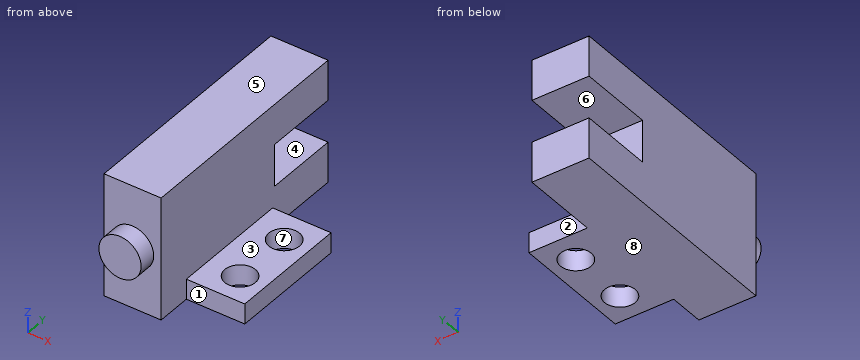
from build123d import *

# Parameters (mm, degrees)
SKETCH_1_W          = 6.5
SKETCH_1_H          = 14
EXTRUDE_1_DEPTH     = 26.5
SKETCH_2_W          = 6.5
SKETCH_2_H          = 4.8
CUT_EXTRUDE_1_DEPTH = 8.5
SKETCH_3_W          = 2.3
SKETCH_3_H          = 13.7
EXTRUDE_2_DEPTH     = 6.65
SKETCH_4_R          = 1.75
CUT_EXTRUDE_2_DEPTH = 6.65
SKETCH_5_R          = 2.4
EXTRUDE_3_DEPTH     = 2


with BuildPart() as part:
    # 草图1 → 凸台-拉伸1 (new body)
    with BuildSketch(Plane(origin=(0, 0, 0), x_dir=(1, 0, 0), z_dir=(0, 1, 0))):
        with Locations((3.25, 7)):
            Rectangle(SKETCH_1_W, SKETCH_1_H)
    extrude(amount=EXTRUDE_1_DEPTH)

    # 草图2 → 切除-拉伸1 (cut)
    with BuildSketch(Plane(origin=(0, 26.5, 0), x_dir=(1, 0, 0), z_dir=(0, 1, 0))):
        with Locations((3.25, 7)):
            Rectangle(SKETCH_2_W, SKETCH_2_H)
    extrude(amount=-CUT_EXTRUDE_1_DEPTH, mode=Mode.SUBTRACT)

    # 草图3 → 凸台-拉伸2 (add)
    with BuildSketch(Plane(origin=(6.5, 0, 0), x_dir=(0, 0, -1), z_dir=(1, 0, 0))):
        with Locations((12.85, 10.85)):
            Rectangle(SKETCH_3_W, SKETCH_3_H)
    extrude(amount=EXTRUDE_2_DEPTH)

    # 草图4 → 切除-拉伸2 (cut)
    with BuildSketch(Plane.XY.offset(-11.7)):
        with Locations((10.25, 14.3)):
            Circle(SKETCH_4_R)
        with Locations((10.25, 7.3)):
            Circle(SKETCH_4_R)
    extrude(amount=-CUT_EXTRUDE_2_DEPTH, mode=Mode.SUBTRACT)

    # 草图5 → 凸台-拉伸3 (add)
    with BuildSketch(Plane.XZ):
        with Locations(Location((3.25, -7, 0), (0, 0, 270))):
            Circle(SKETCH_5_R)
    extrude(amount=EXTRUDE_3_DEPTH)


solid = part.part
Work out the finished part from the listing and answer in its coordinate system (mm). Face numbers are marked on the shaded views. A direction names the side the tool comes from. Give positions to 0.01 mm unless a question says otherwise; leave off trailing zeros. Loops run counter-clockwise (first coordinate to the right, second up) from the corner with the lowest first, then second, coordinate; pieces in that order, holes last. Notation, with made-up numbers: (84, 34) - (105, 34) arc R21 cw to (105, 42) - close; hole circle Ø9 at (-30.5, 39). An arc over 180 degrees is marked (long way). Answer in a Markdown table with one row per item. Add a question column.
Q1. A tool of negligible diameter and unlimited length cuts with its end or side. For the marked faces 1, 2, 3, 4 and 5, from which of +Z, -Z, +X, -X, +Y, -Y can it reach the whole face along a straight path? Write none if from no direction.
Q2. Each of these flat-tipped pins is pushed along its axis until it touches: P1, Ø2.5, axis at x = 10.5, z = -13, coming from the -Y side; P2, Ø1.2, axis at x = 11.5, z = -13, coming from the +Y side; P3, Ø1.4, axis at x = 2.5, z = -7, coming from the +Y side. Where does it stop, or does it pass through?
Q3. The part is cut by section B-B (y = 7.3). Determine the outline of the cut face in (x, z).
Q4. Consider line 1 along Y through (x, z) = (10.25, -12.8); line 2 along Z through (x, y) = (1.5, 19); line 3 along Z through (x, y) = (9.75, 12). Determine where each line is inside the solid, lowest interval first.
Q5. The part is cut by section C-C (z = -7). Determine the outline of the cut face in (x, y).
Q6. The part is cut by section D-D (y = 23.5). Determine the outline of the cut face in (x, z), and give its area (3 significant figures).
Q7. The part is cut by section A-A (x = 10.25). Determine the outline of the cut face in (y, z), and give its area (3 significant figures).
Q8. Determine the mould class of the marked faces 6, 7 and 8 for opening direction Z: released by +Z, released by -Z, zero draft, split by the parting line, or undercut.
Solution:
| question | item | result |
|---|---|---|
| 1 | face 1 | +Z, -Z, +X, -Y |
| 1 | face 2 | +Z, -Z, +X, +Y |
| 1 | face 3 | +Z, +X, +Y, -Y |
| 1 | face 4 | +X, -X, +Y |
| 1 | face 5 | +Z, +X, -X, +Y, -Y |
| 2 | P1 | stops at y = 4 |
| 2 | P2 | stops at y = 17.7 |
| 2 | P3 | stops at y = 18 |
| 3 | outline | (0, -14) - (8.5, -14) - (8.5, -11.7) - (6.5, -11.7) - (6.5, 0) - (0, 0) - close; (12, -14) - (13.15, -14) - (13.15, -11.7) - (12, -11.7) - close |
| 4 | line 1 | y = 4 to 5.55, 9.05 to 12.55, 16.05 to 17.7 |
| 4 | line 2 | z = -14 to -9.4, -4.6 to 0 |
| 4 | line 3 | z = -14 to -11.7 |
| 5 | outline | (0, 0) - (0.85, 0) - (0.85, -2) - (5.65, -2) - (5.65, 0) - (6.5, 0) - (6.5, 18) - (0, 18) - close |
| 6 | outline | (0, -14) - (6.5, -14) - (6.5, -9.4) - (0, -9.4) - close; (0, -4.6) - (6.5, -4.6) - (6.5, 0) - (0, 0) - close |
| 6 | area | 59.8 mm² |
| 7 | outline | (4, -14) - (5.55, -14) - (5.55, -11.7) - (4, -11.7) - close; (9.05, -14) - (12.55, -14) - (12.55, -11.7) - (9.05, -11.7) - close; (16.05, -14) - (17.7, -14) - (17.7, -11.7) - (16.05, -11.7) - close |
| 7 | area | 15.4 mm² |
| 8 | face 6 | undercut |
| 8 | face 7 | zero draft |
| 8 | face 8 | released by -Z |
